from build123d import *

# Parameters (mm, degrees)
SKETCH1_W           = 19.43
SKETCH1_H           = 35.05
BOARD_OUTLINE_DEPTH = 0.79
SKETCH2_R           = 0.405
SKETCH2_R_2         = 0.76
PTH_DEPTH           = 41.083057518


with BuildPart() as part:
    # Sketch1 → Board_Outline (new body)
    with BuildSketch(Plane.XY):
        with Locations((9.715, 17.525)):
            Rectangle(SKETCH1_W, SKETCH1_H)
    extrude(amount=BOARD_OUTLINE_DEPTH)

    # Sketch2 → PTH (cut, through all)
    with BuildSketch(Plane.XY):
        with Locations((18.08, 5.31)):
            Circle(SKETCH2_R)
        with Locations((17.88, 33.32)):
            Circle(SKETCH2_R)
        with Locations(Location((2.64, 8.05, 0), (0, 0, 180))):
            Circle(SKETCH2_R_2)
        with Locations(Location((2.64, 2.03, 0), (0, 0, 180))):
            Circle(SKETCH2_R_2)
        with Locations((18.08, 7.96)):
            Circle(SKETCH2_R)
        with Locations((1.52, 33.32)):
            Circle(SKETCH2_R)
        with Locations((18.08, 1.78)):
            Circle(SKETCH2_R)
    extrude(amount=PTH_DEPTH, mode=Mode.SUBTRACT)


solid = part.part
For this review, take the finished solid that the model builds, in its own axes (mm). Coordinates: 2 decimals unless noted, no trailing zeros. Order: outer loops, then holes, each group sorted by start corner. A loop starts at its lowest first (then second) coordinate and runs counter-clockwise, first axis right, second up. Notation, with made-up numbers: (6, 31) - (40, 31) arc R13 ccw to (40, 55) - close; hole circle Ø5 at (51, 86.25). An arc over 180 degrees is marked (long way). Use one line per item in the form item = value.
Q1. Consider section A-A (y = 5.31). Give the boundary of the cut face in (x, z) (3 decimals), then the cut area to 3 significant figures.
Checked values:
outline = (0, 0) - (17.675, 0) - (17.675, 0.79) - (0, 0.79) - close; (18.485, 0) - (19.43, 0) - (19.43, 0.79) - (18.485, 0.79) - close
area = 14.7 mm2
Q2. Draft analysis for pull direction Y (two halves, no side actions). For faces 1 (the cylindrical face through (1.432, 32.925, 0.389)), 2 (the flat face through (10, 18, 0.79)), state which applies: +Y half, -Y half, draft (parallel to the pull), parting line (faces both ways), or undercut.
Checked values:
face_1 = undercut
face_2 = draft
Q3. For P1, Ø2, axis at x = 2.64, y = 8.05, coming from the -Z side; P2, Ø1.2, axis at x = 2.64, y = 2.03, coming from the -Z side, all flat-tipped, find the tip position at first contact; note any pin that passes through.
Checked values:
P1 = 0
P2 = through
Q4. Consider section C-C (y = 33.32). Give the boundary of the cut face in (x, z) (3 decimals), then the cut area to 3 significant figures.
Checked values:
outline = (0, 0) - (1.115, 0) - (1.115, 0.79) - (0, 0.79) - close; (1.925, 0) - (17.475, 0) - (17.475, 0.79) - (1.925, 0.79) - close; (18.285, 0) - (19.43, 0) - (19.43, 0.79) - (18.285, 0.79) - close
area = 14.1 mm2
Q5. Consider section B-B (x = 2.64). Give the boundary of the cut face in (y, z).
Checked values:
outline = (0, 0) - (1.27, 0) - (1.27, 0.79) - (0, 0.79) - close; (2.79, 0) - (7.29, 0) - (7.29, 0.79) - (2.79, 0.79) - close; (8.81, 0) - (35.05, 0) - (35.05, 0.79) - (8.81, 0.79) - close
Q6. For probe 1 along X at (y, z) = (33.32, 0.3) (3 decimals); probe 2 along Y at (x, z) = (2.75, 0.7); probe 3 along X at (y, z) = (7.96, 0.35) (3 decimals), list the stretches that pass through material, from the lowest coordinate up. Write a range as from..to.
Checked values:
probe_1 = 0..1.115, 1.925..17.475, 18.285..19.43
probe_2 = 0..1.28, 2.78..7.3, 8.8..35.05
probe_3 = 0..1.885, 3.395..17.675, 18.485..19.43
